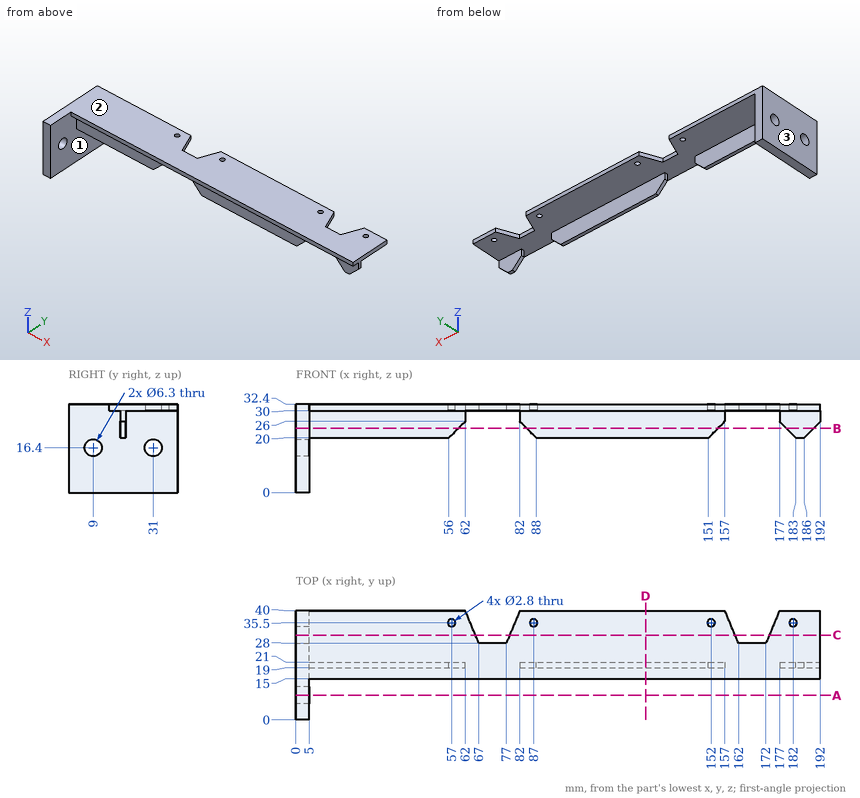
Input: dimensioned drawing with shaded views. Units: mm. Origin: part minimum x, y, z. Coordinates: 2 decimals unless noted, no trailing zeros. Order: outer loops, then holes, each group sorted by start corner. A loop starts at its lowest first (then second) coordinate and runs counter-clockwise, first axis right, second up.
1. Cut plane A-A, the plane y = 9. Return loops of the section in (x, z).
Checked values:
outline: (0, 0) - (5, 0) - (5, 13.25) - (0, 13.25) - close; (0, 19.55) - (5, 19.55) - (5, 32.4) - (0, 32.4) - close
2. Cut plane C-C, the plane y = 31. Return loops of the section in (x, z), plus the area to 3 significant figures.
Checked values:
outline: (0, 0) - (5, 0) - (5, 13.25) - (0, 13.25) - close; (0, 19.55) - (5, 19.55) - (5, 30) - (65.75, 30) - (65.75, 32.4) - (0, 32.4) - close; (78.25, 30) - (160.75, 30) - (160.75, 32.4) - (78.25, 32.4) - close; (173.25, 30) - (192, 30) - (192, 32.4) - (173.25, 32.4) - close
area: 519 mm2
3. Cut plane B-B, the plane z = 23.5. Return loops of the section in (x, y), plus the area to 3 significant figures.
Checked values:
outline: (0, 0) - (5, 0) - (5, 19) - (59.5, 19) - (59.5, 21) - (5, 21) - (5, 40) - (0, 40) - close; (84.5, 19) - (154.5, 19) - (154.5, 21) - (84.5, 21) - close; (179.5, 19) - (189.5, 19) - (189.5, 21) - (179.5, 21) - close
area: 469 mm2
4. Ray query, line 1 along Y through (x, z) = (2.45, 16.4); line 2 along Y through (x, z) = (152, 31); line 3 along Z through (x, y) = (163, 26). Return the intervals inside material, ascending.
Checked values:
line 1: y = 0 to 5.85, 12.15 to 27.85, 34.15 to 40
line 2: y = 15 to 34.1, 36.9 to 40
line 3: z = 30 to 32.4
5. Draft query along X for the marked faces 1, 2 and 3. Return one class per face: +X half, -X half, draft (parallel to the pull), parting line (faces both ways), or undercut.
Checked values:
face 1: +X half
face 2: draft
face 3: -X half
6. Contact query for flat-ended pins moving along their axis: P1, Ø7.5, axis at x = 53, y = 23.5, coming from the -Z side; P2, Ø1, axis at y = 33, z = 23.5, coming from the +X side; P3, Ø3, axis at x = 109.5, z = 23, coming from the +Y side; P4, Ø5, axis at y = 9, z = 16.4, coming from the -X side. Output: stop coordinate, or through.
Checked values:
P1: stops at z = 20
P2: stops at x = 5
P3: stops at y = 21
P4: passes through
7. Cut plane D-D, the plane x = 128. Return loops of the section in (y, z).
Checked values:
outline: (15, 30) - (19, 30) - (19, 20) - (21, 20) - (21, 30) - (40, 30) - (40, 32.4) - (15, 32.4) - close
